For this review, take the finished solid that the model builds, in its own axes (mm). Face numbers are marked on the shaded views. Round coordinates to 2 decimals unless told otherwise and drop trailing zeros. Loops run counter-clockwise (first coordinate to the right, second up) from the corner with the lowest first, then second, coordinate; pieces in that order, holes last.
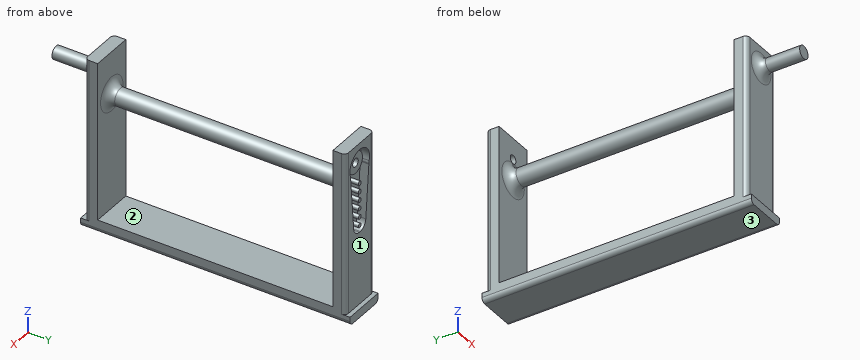
```python
from build123d import *

# Parameters (mm, degrees)
SKETCH1_W             = 10
SKETCH1_H             = 40
BOSS_EXTRUDE1_DEPTH   = 3
CAVITY4_START         = 1
CAVITY4_OUTLINE_R     = 2.5
CAVITY4_OUTLINE_R_2   = 0.5
CAVITY4_DEPTH         = 2
CAVITY4_START_2       = 2
CAVITY4_2_OUTLINE_R   = 2.5
CAVITY4_2_OUTLINE_R_2 = 1
CAVITY4_2_DEPTH       = 1
CUT_EXTRUDE4_START    = -23
SKETCH5_R             = 1
CUT_EXTRUDE4_DEPTH    = 23
SKETCH7_W             = 10
SKETCH7_H             = 3
BOSS_EXTRUDE3_DEPTH   = 55
SKETCH8_R             = 1.5
BOSS_EXTRUDE4_DEPTH   = 10
SKETCH9_W             = 10
SKETCH9_H             = 2
BOSS_EXTRUDE5_DEPTH   = 1
FILLET2_R             = 1
FILLET3_R             = 1
FILLET4_R             = 2
SKETCH10_R            = 2
BOSS_EXTRUDE6_DEPTH   = 55
FILLET5_R             = 2
FILLET6_R             = 1


# Read off the part's stored shape, not the designer's step: Cavity4
with BuildPart() as part:
    # Sketch1 → Boss-Extrude1 (new body)
    with BuildSketch(Plane(origin=(0, 0, 0), x_dir=(1, 0, 0), z_dir=(0, 1, 0))):
        with Locations((1.621359223, -14.684466019)):
            Rectangle(SKETCH1_W, SKETCH1_H)
    boss_extrude1 = extrude(amount=BOSS_EXTRUDE1_DEPTH)

    # Cavity4 outline → Cavity4 (cut)
    with BuildSketch(Plane(origin=(0, 0, 0), x_dir=(1, 0, 0), z_dir=(0, 1, 0)).offset(CAVITY4_START)):
        with BuildLine():
            Line((-0.538748891, -15.509698524), (-1.620990225, -27.847249725))
            ThreePointArc((-1.620990225, -27.847249725), (-1.626727223, -27.934549786), (-1.628640777, -28.022017221))
            Line((-1.628640777, -28.022017221), (-1.628640777, -28.045106388))
            ThreePointArc((-1.628640777, -28.045106388), (-1.65149867, -28.346617733), (-1.719549868, -28.641237163))
            ThreePointArc((-1.719549868, -28.641237163), (1.621359223, -33.184466019), (4.962268314, -28.641237163))
            ThreePointArc((4.962268314, -28.641237163), (4.894217117, -28.346617733), (4.871359223, -28.045106388))
            Line((4.871359223, -28.045106388), (4.871359223, -28.022017221))
            ThreePointArc((4.871359223, -28.022017221), (4.86944567, -27.934549786), (4.863708671, -27.847249725))
            Line((4.863708671, -27.847249725), (3.781467338, -15.509698524))
            ThreePointArc((3.781467338, -15.509698524), (3.14012955, -14.209756728), (1.78911789, -13.684466019))
            Line((1.78911789, -13.684466019), (1.453600557, -13.684466019))
            ThreePointArc((1.453600557, -13.684466019), (0.102588897, -14.209756728), (-0.538748891, -15.509698524))
        make_face()
        with Locations((1.621359223, -29.684466019)):
            Circle(CAVITY4_OUTLINE_R, mode=Mode.SUBTRACT)
        with Locations((1.621359223, -25.184466019)):
            Circle(CAVITY4_OUTLINE_R_2, mode=Mode.SUBTRACT)
        with Locations((1.621359223, -23.184466019)):
            Circle(CAVITY4_OUTLINE_R_2, mode=Mode.SUBTRACT)
        with Locations((1.621359223, -21.184466019)):
            Circle(CAVITY4_OUTLINE_R_2, mode=Mode.SUBTRACT)
        with Locations((1.621359223, -19.184466019)):
            Circle(CAVITY4_OUTLINE_R_2, mode=Mode.SUBTRACT)
        with Locations((1.621359223, -17.184466019)):
            Circle(CAVITY4_OUTLINE_R_2, mode=Mode.SUBTRACT)
        with Locations((1.621359223, -15.184466019)):
            Circle(CAVITY4_OUTLINE_R_2, mode=Mode.SUBTRACT)
    extrude(amount=CAVITY4_DEPTH, mode=Mode.SUBTRACT)

    # Cavity4 2 outline → Cavity4 2 (cut)
    with BuildSketch(Plane(origin=(0, 0, 0), x_dir=(1, 0, 0), z_dir=(0, 1, 0)).offset(CAVITY4_START_2)):
        with Locations((1.621359223, -29.684466019)):
            Circle(CAVITY4_2_OUTLINE_R)
        with Locations((1.621359223, -29.684466019)):
            Circle(CAVITY4_2_OUTLINE_R_2, mode=Mode.SUBTRACT)
    extrude(amount=CAVITY4_2_DEPTH, mode=Mode.SUBTRACT)

    # Sketch5 → Cut-Extrude4 (cut)
    with BuildSketch(Plane(origin=(0, 3, 0), x_dir=(1, 0, 0), z_dir=(0, 1, 0)).offset(CUT_EXTRUDE4_START)):
        with Locations(Location((1.621359223, -29.684466019, 0), (0, 0, 270))):
            Circle(SKETCH5_R)
    extrude(amount=CUT_EXTRUDE4_DEPTH, mode=Mode.SUBTRACT)

    # Sketch7 → Boss-Extrude3 (add)
    with BuildSketch(Plane.XZ):
        with Locations((1.621359223, -3.815533981)):
            Rectangle(SKETCH7_W, SKETCH7_H)
    extrude(amount=BOSS_EXTRUDE3_DEPTH)

    # Mirror1: Boss-Extrude1 across plane
    add(boss_extrude1.mirror(Plane(origin=(0, -27.5, 0), x_dir=(0, 0, 1), z_dir=(0, -1, 0))))

    # Sketch8 → Boss-Extrude4 (add)
    with BuildSketch(Plane.XZ.offset(58)):
        with Locations(Location((1.621359223, 29.684466019, 0), (0, 0, 270))):
            Circle(SKETCH8_R)
    extrude(amount=BOSS_EXTRUDE4_DEPTH)

    # Sketch9 → Boss-Extrude5 (add)
    with BuildSketch(Plane.XZ.offset(58)):
        with Locations((1.621359223, -4.315533981)):
            Rectangle(SKETCH9_W, SKETCH9_H)
    boss_extrude5 = extrude(amount=BOSS_EXTRUDE5_DEPTH)

    # Mirror2: Boss-Extrude5 across plane
    add(boss_extrude5.mirror(Plane(origin=(0, -27.5, 0), x_dir=(0, 0, 1), z_dir=(0, -1, 0))))

    # Fillet2
    fillet2_edges = [part.edges().sort_by_distance(p)[0] for p in [
        (6.621359223, 3, 15.684466019),
        (6.621359223, -58, 15.684466019),
    ]]
    fillet(fillet2_edges, radius=FILLET2_R)

    # Fillet3
    fillet3_edges = [part.edges().sort_by_distance(p)[0] for p in [
        (-3.378640777, -58, 15.684466019),
        (-3.378640777, 3, 15.684466019),
    ]]
    fillet(fillet3_edges, radius=FILLET3_R)

    # Fillet4
    fillet4_edges = [part.edges().sort_by_distance(p)[0] for p in [
        (1.621359223, -58, 31.184466019),
    ]]
    fillet(fillet4_edges, radius=FILLET4_R)

    # Sketch10 → Boss-Extrude6 (add)
    with BuildSketch(Plane.XZ):
        with Locations(Location((1.621359223, 24.751865002, 0), (0, 0, 90))):
            Circle(SKETCH10_R)
    extrude(amount=BOSS_EXTRUDE6_DEPTH)

    # Fillet5
    fillet5_edges = [part.edges().sort_by_distance(p)[0] for p in [
        (1.621359223, -55, 22.751865002),
        (1.621359223, 0, 22.751865002),
    ]]
    fillet(fillet5_edges, radius=FILLET5_R)

    # Fillet6
    fillet6_edges = [part.edges().sort_by_distance(p)[0] for p in [
        (-3.378640777, -27.5, -5.315533981),
        (6.621359223, -27.5, -5.315533981),
    ]]
    fillet(fillet6_edges, radius=FILLET6_R)


solid = part.part
```
(1) Add section A-A (z = 9). Give the boundary of the cut face in (x, y), plus the area to 3 significant figures.
(2) Add section B-B (y = -41.5). Give the boundary of the cut face in (x, z), plus the area to 3 significant figures.
(3) The part is to be moulded in two halves that separate along Z. For the marked faces 1, 2 and 3, say which applies: pulls with the +Z half, pulls with the -Z half, needs draft (parallel to the pull), parting line crosses it, or undercut.
(4) For L1, parallel to Y at x = 4.25, z = 15.5; L2, parallel to Y at x = 2.5, z = 33; L3, parallel to Z at x = 0.75, y = -9.5, list the stretches that pass through material, from the lowest coordinate up.
(5) Insertion check: pin 1 Ø1.5 at (y, z) = (-20, 25) entering from +X; pin 2 Ø2 at (x, z) = (1, 6) entering from +Y; pin 3 Ø6 at (x, z) = (3.5, 15.5) entering from -Y. Each pin has a flat end and moves straight along its axis. Give the tip position at first contact, or say it passes through.
Outcome:
1. outline: (-3.38, -57) arc R1 ccw to (-2.38, -58) - (5.62, -58) arc R1 ccw to (6.62, -57) - (6.62, -55) - (-3.38, -55) - close; (-3.38, 0) - (6.62, 0) - (6.62, 2) arc R1 ccw to (5.62, 3) - (-2.38, 3) arc R1 ccw to (-3.38, 2) - close
1. area: 59.1 mm2
2. outline: (-3.38, -4.32) arc R1 ccw to (-2.38, -5.32) - (5.62, -5.32) arc R1 ccw to (6.62, -4.32) - (6.62, -2.32) - (-3.38, -2.32) - close; circle Ø4 at (1.62, 24.75)
2. area: 42.1 mm2
3. face 1: needs draft
3. face 2: undercut
3. face 3: pulls with the -Z half
4. L1: y = -58 to -55, 0 to 3
4. L2: y = -58 to -55, 0 to 1
4. L3: z = -5.32 to -2.32, 22.95 to 26.55
5. pin 1: stops at x = 3.62
5. pin 2: stops at y = 3
5. pin 3: stops at y = -58
